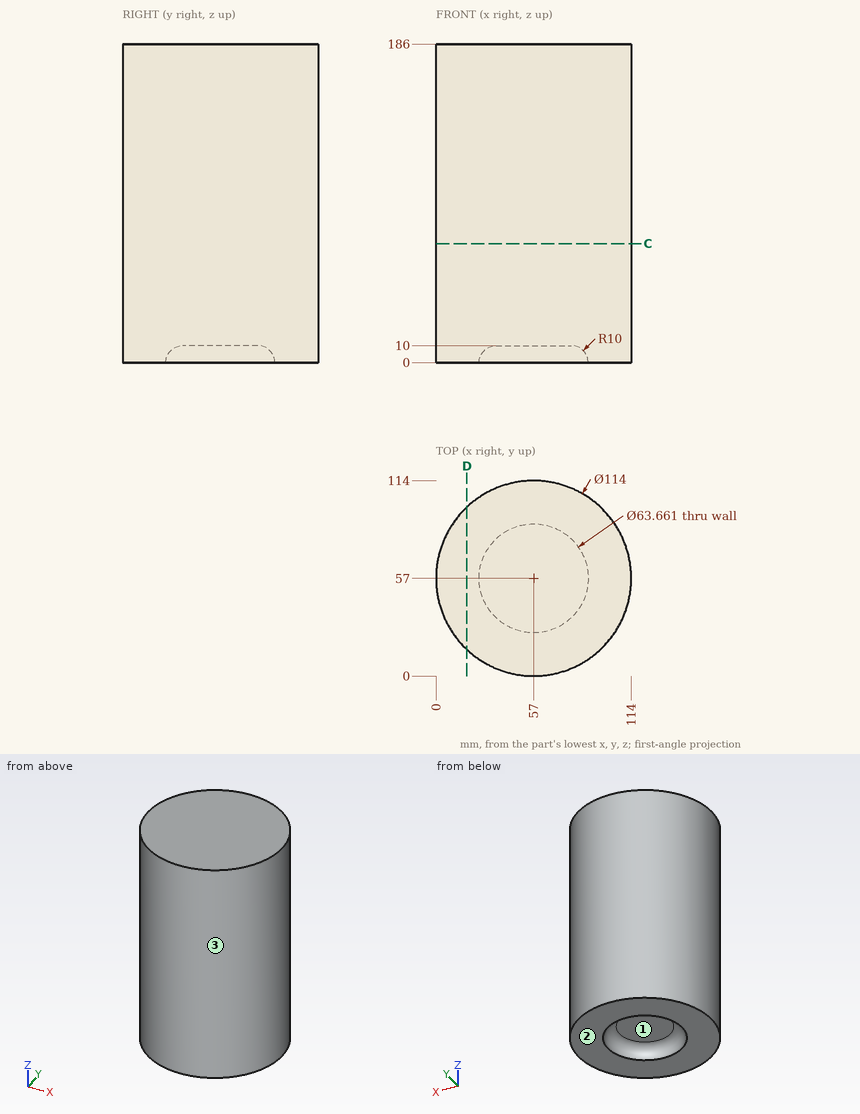
Here's the drawing with two shaded views (mm, measured from the low corner). I have some questions. Give positions to 0.01 mm unless a question says otherwise; leave off trailing zeros. Loops run counter-clockwise (first coordinate to the right, second up) from the corner with the lowest first, then second, coordinate; pieces in that order, holes last. Notation, with made-up numbers: M 33.25,11.25 L 37.25,11.25 A10 cw 37.25,17.25 Z; hole C 52.25,73 d3. An arc over 180 degrees is marked long. Answer in a Markdown table with one row per item.
1. For pin 1 Ø5 at (y, z) = (68.5, 48) entering from +X (3 decimals); pin 2 Ø10 at (y, z) = (17, 150.5) entering from +X; pin 3 Ø3 at (x, z) = (16.5, 69.5) entering from -Y, each with a flat end and sliding along its axis, tell me the tip position at first contact or that it passes through.
Taken from the geometry:
| item | result |
|---|---|
| pin 1 | stops at x = 113.285 |
| pin 2 | stops at x = 101.99 |
| pin 3 | stops at y = 15.43 |
2. Suppose I cut it at C-C on z = 69.5. Write out the boundary of the cut face in (x, y), plus the area to 3 significant figures.
Taken from the geometry:
| item | result |
|---|---|
| outline | C 57,57 d114 |
| area | 10,200 mm² |
3. If I drill on line 1 along Z through (x, y) = (70, 48); line 2 along Y through (x, z) = (57, 0.05); line 3 along X through (y, z) = (20, 8.5), over which ranges is the centre line in solid material (lowest first)?
Taken from the geometry:
| item | result |
|---|---|
| line 1 | z = 10 to 186 |
| line 2 | y = 0 to 25.17, 88.83 to 114 |
| line 3 | x = 13.64 to 100.36 |
4. Thinking about a two-plate mould opening in Y: for the marked faces 1, 2 and 3, which applies, released by +Y, released by -Y, zero draft, split by the parting line, or undercut?
Taken from the geometry:
| item | result |
|---|---|
| face 1 | undercut |
| face 2 | zero draft |
| face 3 | split by the parting line |
5. Suppose I cut it at D-D on x = 18. Write out the boundary of the cut face in (y, z).
Taken from the geometry:
| item | result |
|---|---|
| outline | M 15.43,0 L 98.57,0 L 98.57,186 L 15.43,186 Z |
